Build history of the part. All positions in model axes, mm. Face numbers are marked on the shaded views. A direction names the side the tool comes from. Give positions to 0.01 mm unless a question says otherwise; leave off trailing zeros. Order: outer loops, then holes, each group sorted by start corner. A loop starts at its lowest first (then second) coordinate and runs counter-clockwise, first axis right, second up. Notation, with made-up numbers: (39, -23.75) - (78, -23.75) arc R26 cw to (78, -2.75) - close; hole circle Ø9 at (6, -14.5). An arc over 180 degrees is marked (long way). Write each question's results on one line, items separated by ' | '. Start each with the question number.
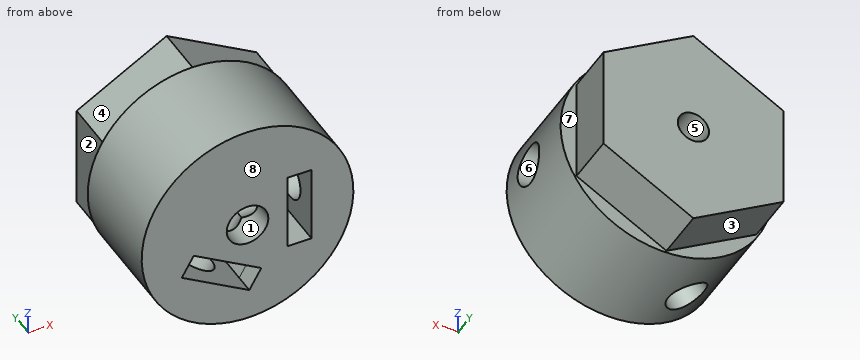
from build123d import *

# Parameters (mm, degrees)
SKETCH_1_R                           = 10.18
EXTRUDE_355_DEPTH                    = 10
EXTRUDE_479_DEPTH                    = 5
SKETCH_3_R                           = 2
CUT_EXTRUDE_578_DEPTH                = 8.6
SKETCH_4_W                           = 2.3
SKETCH_4_H                           = 7.5
CUT_EXTRUDE_807_DEPTH                = 8
SKETCH_5_R                           = 2
CUT_EXTRUDE_1_DEPTH                  = 23.923204401
CUT_EXTRUDE_1_DIRECTION_2_REACH      = 24.923
CUT_EXTRUDE_1_DIRECTION_2_END_RADIUS = 2
SKETCH_6_R                           = 2
CUT_EXTRUDE_2_DEPTH                  = 24.540700338
CUT_EXTRUDE_2_DIRECTION_2_REACH      = 25.541
CUT_EXTRUDE_2_DIRECTION_2_END_RADIUS = 2
CUT_EXTRUDE_1_2_DEPTH                = 2.3
CUT_EXTRUDE_2_2_DEPTH                = 2.3
SKETCH_9_R                           = 1.5
CUT_EXTRUDE_7_DEPTH                  = 21.790978983


with BuildPart() as part:
    # Эскиз1 → Extrude 355 (new body)
    with BuildSketch(Plane(origin=(0, 0, 0), x_dir=(1, 0, 0), z_dir=(0, 1, 0))):
        with Locations(Location((0, 0, 0), (0, 0, 270))):
            Circle(SKETCH_1_R)
    extrude(amount=EXTRUDE_355_DEPTH)

    # Эскиз2 → Extrude 479 (add)
    with BuildSketch(Plane(origin=(0, 10, 0), x_dir=(1, 0, 0), z_dir=(0, 1, 0))):
        Polygon((0, 9.988159657), (-8.65, 4.994079828), (-8.65, -4.994079828), (0, -9.988159657), (8.65, -4.994079828), (8.65, 4.994079828), align=None)
    extrude(amount=EXTRUDE_479_DEPTH)

    # Эскиз3 → Cut-Extrude 578 (cut)
    with BuildSketch(Plane.XZ):
        with Locations(Location((0, 0, 0), (0, 0, 270))):
            Circle(SKETCH_3_R)
    extrude(amount=-CUT_EXTRUDE_578_DEPTH, mode=Mode.SUBTRACT)

    # Эскиз4 → Cut-Extrude 807 (cut)
    with BuildSketch(Plane.XZ):
        Polygon((-5.172595264, -1.459197805), (1.322595264, -5.209197805), (0.172595264, -7.201056233), (-6.322595264, -3.451056233), align=None)
        with Locations((5, 0)):
            Rectangle(SKETCH_4_W, SKETCH_4_H)
    extrude(amount=-CUT_EXTRUDE_807_DEPTH, mode=Mode.SUBTRACT)

    # Эскиз5 → Cut-Extrude 1 (cut)
    with BuildSketch(Plane(origin=(3.85, 0, 0), x_dir=(0, 0, -1), z_dir=(1, 0, 0))):
        with Locations(Location((0, 4.041451884, 0), (0, 0, 270))):
            Circle(SKETCH_5_R)
    extrude(amount=CUT_EXTRUDE_1_DEPTH, mode=Mode.SUBTRACT)

    # Cut-Extrude 1 direction 2: up to this cylinder (the profile starts outside it)
    cut_extrude_1_direction_2_end = Plane(origin=(0, 4.041452, 0), z_dir=(0, -1, 0)) * Cylinder(CUT_EXTRUDE_1_DIRECTION_2_END_RADIUS, 54.846, mode=Mode.PRIVATE)
    # Эскиз5 → Cut-Extrude 1 direction 2 (cut, up to the surface)
    with BuildSketch(Plane(origin=(3.85, 0, 0), x_dir=(0, 0, -1), z_dir=(1, 0, 0)), mode=Mode.PRIVATE) as cut_extrude_1_direction_2_sk1:
        with Locations(Location((0, 4.041451884, 0), (0, 0, 270))):
            Circle(SKETCH_5_R)
    cut_extrude_1_direction_2_tool1 = extrude(cut_extrude_1_direction_2_sk1.sketch, amount=-CUT_EXTRUDE_1_DIRECTION_2_REACH, mode=Mode.PRIVATE) - cut_extrude_1_direction_2_end
    add(cut_extrude_1_direction_2_tool1.solids().sort_by_distance((3.85, 4.041452, 0))[0], mode=Mode.SUBTRACT)

    # Эскиз6 → Cut-Extrude 2 (cut)
    with BuildSketch(Plane(origin=(-1.925, 0, -3.334197805), x_dir=(-0.8660254037844363, 0, 0.5000000000000042), z_dir=(-0.5000000000000042, 0, -0.8660254037844363))):
        with Locations(Location((0, 4.041451884, 0), (0, 0, 180))):
            Circle(SKETCH_6_R)
    extrude(amount=CUT_EXTRUDE_2_DEPTH, mode=Mode.SUBTRACT)

    # Cut-Extrude 2 direction 2: up to this cylinder (the profile starts outside it)
    cut_extrude_2_direction_2_end = Plane(origin=(0, 4.041452, 0), z_dir=(0, -1, 0)) * Cylinder(CUT_EXTRUDE_2_DIRECTION_2_END_RADIUS, 56.082, mode=Mode.PRIVATE)
    # Эскиз6 → Cut-Extrude 2 direction 2 (cut, up to the surface)
    with BuildSketch(Plane(origin=(-1.925, 0, -3.334197805), x_dir=(-0.8660254037844363, 0, 0.5000000000000042), z_dir=(-0.5000000000000042, 0, -0.8660254037844363)), mode=Mode.PRIVATE) as cut_extrude_2_direction_2_sk1:
        with Locations(Location((0, 4.041451884, 0), (0, 0, 180))):
            Circle(SKETCH_6_R)
    cut_extrude_2_direction_2_tool1 = extrude(cut_extrude_2_direction_2_sk1.sketch, amount=-CUT_EXTRUDE_2_DIRECTION_2_REACH, mode=Mode.PRIVATE) - cut_extrude_2_direction_2_end
    add(cut_extrude_2_direction_2_tool1.solids().sort_by_distance((-1.925, 4.041452, -3.334198))[0], mode=Mode.SUBTRACT)

    # Эскиз7 → Cut-Extrude 1 2 (cut)
    with BuildSketch(Plane(origin=(3.85, 0, 0), x_dir=(0, 0, -1), z_dir=(1, 0, 0))):
        Polygon((-3.75, 1.876388375), (0, -0.288675135), (3.75, 1.876388375), (3.75, 6.206515394), (0, 8.371578903), (-3.75, 6.206515394), align=None)
    extrude(amount=CUT_EXTRUDE_1_2_DEPTH, mode=Mode.SUBTRACT)

    # Эскиз8 → Cut-Extrude 2 2 (cut)
    with BuildSketch(Plane(origin=(-1.925, 0, -3.334197805), x_dir=(-0.8660254037844363, 0, 0.5000000000000042), z_dir=(-0.5000000000000042, 0, -0.8660254037844363))):
        Polygon((0, 8.371578903), (-3.75, 6.206515394), (-3.75, 1.876388375), (0, -0.288675135), (3.75, 1.876388375), (3.75, 6.206515394), align=None)
    extrude(amount=CUT_EXTRUDE_2_2_DEPTH, mode=Mode.SUBTRACT)

    # Эскиз9 → Вырез-Вытянуть7 (cut, through all)
    with BuildSketch(Plane(origin=(0, 15, 0), x_dir=(1, 0, 0), z_dir=(0, 1, 0))):
        with Locations(Location((0, 0, 0), (0, 0, 270))):
            Circle(SKETCH_9_R)
    extrude(amount=-CUT_EXTRUDE_7_DEPTH, mode=Mode.SUBTRACT)


solid = part.part
Item 1: Cut at C-C, the plane x = 7.5. List the corners of the cut face in (y, z), then the cut area to 3 significant figures.
Item 2: Which spindle directions (+Z, -Z, +X, -X, +Y, -Y) get a long thin tool onto all of the face, cutting with end or side? Do the marked faces 1, 2, 3 and 4. Say none if no direction does.
Item 3: Cut at D-D, the plane z = 5.5. List the corners of the cut face in (x, y), then the cut area to 3 significant figures.
Item 4: Cut at B-B, the plane y = 3.5. List the corners of the cut face in (x, z).
Item 5: Probe line 1 along X through (y, z) = (14.5, -2); line 2 along Y through (x, z) = (-9, -4); line 3 along Z through (x, y) = (-5.25, 4.25). List the from-to ranges inside material, lowest first. Write a range as from..to.
Item 6: Cut at A-A, the plane y = 11.75. List the corners of the cut face in (x, z), then the cut area to 3 significant figures.
Item 7: Two-plate mould, pull along Y, no slides. Class the marked faces 5, 6, 7 and 8: +Y half, -Y half, draft (parallel to the pull), parting line (faces both ways), or undercut.
Item 8: Flat gauge pins, fed straight in: pin 1 Ø1.5 at (y, z) = (13.5, 2.5) entering from -X; pin 2 Ø1 at (x, y) = (3.5, 10) entering from +Z; pin 3 Ø8 at (y, z) = (7, -7.5) entering from +X. Where does each tip first touch, or does it go through?
Values found:
1) outline: (0, -6.88) - (10, -6.88) - (10, -5.66) - (15, -5.66) - (15, 5.66) - (10, 5.66) - (10, 6.88) - (0, 6.88) - close; hole circle Ø4 at (4.04, 0) | area: 182 mm2
2) face 1: -Y | face 2: +Z, -Z, -X, +Y | face 3: -Z, -X, +Y | face 4: +Z, -X, +Y
3) outline: (-8.57, 0) - (8.57, 0) - (8.57, 10) - (7.77, 10) - (7.77, 15) - (-7.77, 15) - (-7.77, 10) - (-8.57, 10) - close | area: 249 mm2
4) outline: (-6.67, -7.69) - (-4.74, -4.36) - (-6.32, -3.45) - (-5.17, -1.46) - (-3.59, -2.37) - (-1.94, 0.49) arc R2 cw to (0.54, 1.93) - (3.85, 1.93) - (3.85, 3.75) - (6.15, 3.75) - (6.15, 1.93) - (10, 1.93) arc R10.18 ccw (long way) to start; (-3.33, -9.62) arc R10.18 ccw to (10, -1.93) - (6.15, -1.93) - (6.15, -3.75) - (3.85, -3.75) - (3.85, -1.93) - (1.11, -1.93) - (-0.26, -4.3) - (1.32, -5.21) - (0.17, -7.2) - (-1.41, -6.29) - close
5) line 1: x = -8.65..8.65 | line 2: y = 0..10 | line 3: z = -5.12..-4.07, -1.59..8.72
6) outline: (-8.65, -4.99) - (0, -9.99) - (8.65, -4.99) - (8.65, 4.99) - (0, 9.99) - (-8.65, 4.99) - close; hole circle Ø3 at (0, 0) | area: 252 mm2
7) face 5: draft | face 6: undercut | face 7: +Y half | face 8: -Y half
8) pin 1: stops at x = -8.65 | pin 2: stops at z = 9.73 | pin 3: stops at x = 9.56
